For this review, take the finished solid that the model builds, in its own axes (mm). Round coordinates to 2 decimals unless told otherwise and drop trailing zeros. Write each loop counter-clockwise with the first axis right and the second up, starting at its lowest first coordinate (ties: lowest second). Pieces come first, ordered by that corner, then holes. Notation, with made-up numbers: (54, 78) -> (72, 78) arc R14 cw to (72, 96) -> close; hole circle Ø2 at (-37, 81.25). An arc over 180 degrees is marked (long way). Answer as CSV lines item,"result". Start each with the question number.
Item 1: Take a section at B-B on x = 18. Give the boundary of the cut face in (y, z).
Item 2: Take a section at C-C on x = -10. Give the boundary of the cut face in (y, z).
Item 3: Wall thickness on probe 1 along X at (y, z) = (0, 0.8); probe 2 along Y at (x, z) = (-10.5, 0.65); probe 3 along Z at (x, y) = (-18.5, -1.25): over which ranges is each line inside the solid? List them lowest first. Write a range as from..to.
Item 4: For pin 1 Ø7 at (x, y) = (18.15, 0) entering from -Z; pin 2 Ø1.9 at (x, y) = (-10, 0.5) entering from -Z, all flat-tipped, find the tip position at first contact; note any pin that passes through.
Item 5: Take a section at A-A on y = 0. Give the boundary of the cut face in (x, z).
```python
from build123d import *

# Parameters (mm, degrees)
F0_W     = 50.8
F0_H     = 25.4
F1_DEPTH = 5.08
F2_R     = 3.175
F2_R_2   = 3.1623
F2_R_3   = 3.1496
F2_R_4   = 3.1369
F2_R_5   = 3.1242
F3_DEPTH = 1.6002


with BuildPart() as f1:
    # F0 (on Top) → F1 (new body)
    with BuildSketch(Plane.XY):
        Rectangle(F0_W, F0_H)
    extrude(amount=F1_DEPTH)

    # F2 (on face) → F3 (cut)
    with BuildSketch(Plane(origin=(0, 0, 0), x_dir=(1, 0, 0), z_dir=(0, 0, -1))):
        with Locations((-19.073904, 0)):
            Circle(F2_R)
        with Locations((-10.289737, 0)):
            Circle(F2_R_2)
        with Locations((-1.183511, 0)):
            Circle(F2_R_3)
        with Locations((8.620071, 0)):
            Circle(F2_R_4)
        with Locations((18.153338, 0)):
            Circle(F2_R_5)
    extrude(amount=-F3_DEPTH, mode=Mode.SUBTRACT)


solid = f1.part
```
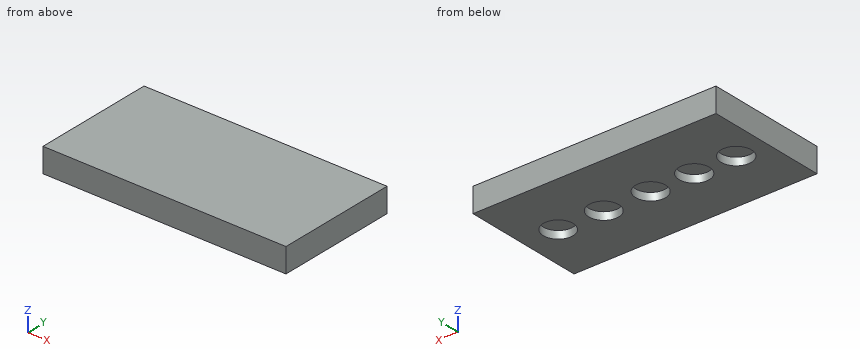
Output values:
1,outline,"(-12.7, 0) -> (-3.12, 0) -> (-3.12, 1.6) -> (3.12, 1.6) -> (3.12, 0) -> (12.7, 0) -> (12.7, 5.08) -> (-12.7, 5.08) -> close"
2,outline,"(-12.7, 0) -> (-3.15, 0) -> (-3.15, 1.6) -> (3.15, 1.6) -> (3.15, 0) -> (12.7, 0) -> (12.7, 5.08) -> (-12.7, 5.08) -> close"
3,probe 1,"x = -25.4..-22.25, -15.9..-13.45, -7.13..-4.33, 1.97..5.48, 11.76..15.03, 21.28..25.4"
3,probe 2,"y = -12.7..-3.16, 3.16..12.7"
3,probe 3,"z = 1.6..5.08"
4,pin 1,"stops at z = 0"
4,pin 2,"stops at z = 1.6"
5,outline,"(-25.4, 0) -> (-22.25, 0) -> (-22.25, 1.6) -> (-15.9, 1.6) -> (-15.9, 0) -> (-13.45, 0) -> (-13.45, 1.6) -> (-7.13, 1.6) -> (-7.13, 0) -> (-4.33, 0) -> (-4.33, 1.6) -> (1.97, 1.6) -> (1.97, 0) -> (5.48, 0) -> (5.48, 1.6) -> (11.76, 1.6) -> (11.76, 0) -> (15.03, 0) -> (15.03, 1.6) -> (21.28, 1.6) -> (21.28, 0) -> (25.4, 0) -> (25.4, 5.08) -> (-25.4, 5.08) -> close"
